Part model, mm, in its own coordinate system. A direction names the side the tool comes from. Coordinates: 2 decimals unless noted, no trailing zeros. Loops run counter-clockwise (first coordinate to the right, second up) from the corner with the lowest first, then second, coordinate; pieces in that order, holes last. Notation, with made-up numbers: M 78.25,2.5 L 92.25,2.5 A28 cw 92.25,27.5 Z; hole C 55,76 d5. An arc over 180 degrees is marked long. Use a Markdown table: item, result. Add a question column.
1) Pull direction Y, two halves, no side cores. Call faces 3 (the flat face through (-22, 0, -12)), 4 (the flat face through (-31, 16.675, -12)), 5 (the flat face through (-44.45, 9, -12)): released by +Y, released by -Y, zero draft, split by the parting line, or undercut.
2) Band-saw the part on C-C (y = 11.5). List the corners of the cut face in (x, z), plus the area to 3 significant figures.
3) Tool access for faces 1 (the flat face through (-22, 9, 0)), 2 (the flat face through (-43.656, 9, -12)): list every direction of +Z, -Z, +X, -X, +Y, -Y with a clear straight run to the whole face (end or side of a thin tool).
4) Band-saw the part on B-B (z = -1.25). List the corners of the cut face in (x, y), plus the area to 3 significant figures.
5) Band-saw the part on A-A (x = -34.5). List the corners of the cut face in (y, z).
6) Wall check: probe 1 along Y at (x, z) = (-39, -7.5); probe 2 along Z at (x, y) = (-42, 2.25); probe 3 along X at (y, z) = (14, -14.5). Give the ranges that are in metal, low to high. Write a range as from..to.
Autodesk Inventor part; units mm, degrees
ref_plane "YZ Plane" through (0, 0, 0) normal (1, 0, 0) x (0, 1, 0)
ref_plane "XZ Plane" through (0, 0, 0) normal (0, 1, 0) x (-1, 0, 0)
ref_plane "XY Plane" through (0, 0, 0) normal (0, 0, 1) x (1, 0, 0)
sketch "Sketch1" plane through (0, 0, 0) normal (0, 1, 0) x (-1, 0, 0)
  line L0 (0, 0) -> (44.45, 0)
  line L1 (44.45, 0) -> (44.45, -23.8125)
  line L2 (44.45, -23.8125) -> (0, -23.8125)
  line L3 (0, -23.8125) -> (0, 0)
  dimension "d0" = 44.45
  dimension "d1" = 23.8125
extrude "Extrusion1" add sketch "Sketch1" along normal blind 1.5875
sketch "Sketch2" plane through (0, 1.5875, 0) normal (0, 1, 0) x (1, 0, 0)
  line L0 (-44.45, 0) -> (0, 0)
  line L1 (0, 0) -> (0, 0.7937)
  line L2 (0, 0.7937) -> (-0.7938, 0.7937)
  line L3 (-44.45, 23.8125) -> (-44.45, 0)
  line L4 (-44.45, 23.8125) -> (-44.45, 23.0187)
  line L5 (-44.45, 23.0187) -> (-43.6563, 23.0187)
  line L6 (-0.7938, 0.7937) -> (-43.6563, 0.7937)
  line L7 (-43.6563, 0.7937) -> (-43.6563, 23.0187)
  line L8 (-43.6563, 23.0187) -> (-0.7938, 23.0187)
  line L9 (-44.45, 23.8125) -> (0, 23.8125)
  line L10 (0, 0) -> (-44.45, 0)
  line L11 (-44.45, 0) -> (-44.45, 23.8125)
  line L12 (-0.7938, 23.0187) -> (0, 23.0187)
  line L13 (0, 0) -> (0, 23.8125)
  line L14 (0, 23.0187) -> (0, 23.8125)
  dimension "d4" = 0.7937
  dimension "d5" = 0.7937
  dimension "d6" = 0.7937
  dimension "d7" = 0.7937
extrude "Extrusion3" add sketch "Sketch2" along normal blind 15.875 contours L3 L5 L7 L6 L2 L1 L0 | L3 L9 L13 L12 L8 L5
sketch "Sketch3" plane through (-43.6563, 1.5875, -0.7937) normal (1, 0, 0) x (0, 0, -1)
  line L0 (0, 15.875) -> (22.225, 15.875)
  line L1 (22.225, 15.875) -> (0, 15.875)
  line L2 (0, 15.875) -> (0, 15.0876)
  line L3 (0, 15.0876) -> (22.225, 15.0876)
  line L4 (22.225, 15.0876) -> (22.225, 15.875)
  point P0 (-0.7937, -1.5875)
  dimension "d12" = 0.7874
extrude "Extrusion4" add sketch "Sketch3" along normal blind 25.4
properties part number "RTCcase"
Entries:
| question | item | result |
|---|---|---|
| 1 | face 3 | released by -Y |
| 1 | face 4 | undercut |
| 1 | face 5 | zero draft |
| 2 | outline | M -44.45,-23.81 L 0,-23.81 L 0,-23.02 L -43.66,-23.02 L -43.66,-0.79 L 0,-0.79 L 0,0 L -44.45,0 Z |
| 2 | area | 88.2 mm2 |
| 3 | face 1 | +Z, +X, -X, +Y, -Y |
| 3 | face 2 | +X |
| 4 | outline | M -44.45,0 L 0,0 L 0,1.59 L -43.66,1.59 L -43.66,16.68 L -18.26,16.68 L -18.26,17.46 L -44.45,17.46 Z |
| 4 | area | 103 mm2 |
| 5 | outline | M 0,-23.81 L 17.46,-23.81 L 17.46,0 L 0,0 Z; hole M 1.59,-23.02 L 16.68,-23.02 L 16.68,-0.79 L 1.59,-0.79 Z |
| 6 | probe 1 | 0..1.59, 16.68..17.46 |
| 6 | probe 2 | -23.81..-23.02, -0.79..0 |
| 6 | probe 3 | -44.45..-43.66 |
